For this review, take the finished solid that the model builds, in its own axes (mm). Face numbers are marked on the shaded views. A direction names the side the tool comes from. Coordinates: 2 decimals unless noted, no trailing zeros. Write each loop counter-clockwise with the first axis right and the second up, starting at its lowest first coordinate (ties: lowest second). Pieces come first, ordered by that corner, then holes. Notation, with made-up numbers: (-8.75, 66.5) - (38.25, 66.5) arc R15 cw to (38.25, 93.5) - close; hole circle Ø4 at (-37, 3.25). An arc over 180 degrees is marked (long way). Write each question's results on one line, items separated by ' | '.
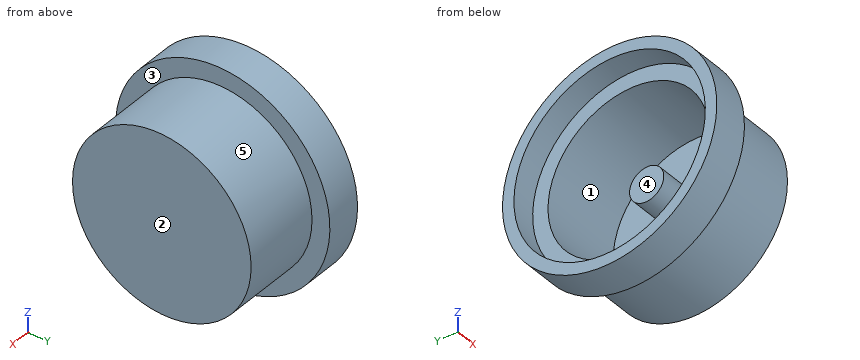
from build123d import *

# Parameters (mm, degrees)
SPUR_START             = 15.199213342
SPUR_GEAR_AM_OUTLINE_R = 1.5
SPUR_GEAR_AM_DEPTH     = 12
SKETCH9_R              = 1.5
BOSS_EXTRUDE1_DEPTH    = 12
SKETCH10_R             = 2.874
BOSS_EXTRUDE2_DEPTH    = 10
SKETCH11_R             = 15
BOSS_EXTRUDE3_DEPTH    = 1
SKETCH12_R             = 15
SKETCH12_R_2           = 13.5
BOSS_EXTRUDE4_DEPTH    = 13
SKETCH13_R             = 18
SKETCH13_R_2           = 13.5
BOSS_EXTRUDE5_DEPTH    = 1.9
SKETCH14_R             = 18
SKETCH14_R_2           = 16.075
BOSS_EXTRUDE6_DEPTH    = 4
SKETCH17_R             = 4
CUT_EXTRUDE2_DEPTH     = 41.416963439
SKETCH19_R             = 2.874
BOSS_EXTRUDE7_DEPTH    = 10


# Read off the part's stored shape, not the designer's step: spur gear_am
with BuildPart() as part:
    # spur gear_am outline → spur gear_am (new body)
    with BuildSketch(Plane.YZ.offset(SPUR_START)):
        with BuildLine():
            ThreePointArc((2.747947228, -4.643773619), (2.654088149, -4.687486435), (2.561391914, -4.733613923))
            ThreePointArc((2.561391914, -4.733613923), (2.561783739, -5.337982285), (2.816889806, -5.88587111))
            ThreePointArc((2.816889806, -5.88587111), (2.597713415, -6.044378226), (2.394409068, -6.222788256))
            ThreePointArc((2.394409068, -6.222788256), (1.9170234, -5.852161498), (1.327895004, -5.717294884))
            ThreePointArc((1.327895004, -5.717294884), (1.262297175, -5.797402699), (1.198794721, -5.879181519))
            ThreePointArc((1.198794721, -5.879181519), (1.461373347, -6.423528591), (1.928936024, -6.806472991))
            ThreePointArc((1.928936024, -6.806472991), (1.800238579, -7.04438004), (1.694476903, -7.293332374))
            ThreePointArc((1.694476903, -7.293332374), (1.103558354, -7.166539081), (0.514255579, -7.300641692))
            ThreePointArc((0.514255579, -7.300641692), (0.489911456, -7.401278171), (0.468180222, -7.502511024))
            ThreePointArc((0.468180222, -7.502511024), (0.940938733, -7.879022193), (1.528351497, -8.021175333))
            ThreePointArc((1.528351497, -8.021175333), (1.515623105, -8.291361907), (1.528351497, -8.56154848))
            ThreePointArc((1.528351497, -8.56154848), (0.940938733, -8.70370162), (0.468180222, -9.080212789))
            ThreePointArc((0.468180222, -9.080212789), (0.489911456, -9.181445642), (0.514255579, -9.28208212))
            ThreePointArc((0.514255579, -9.28208212), (1.103558354, -9.416184732), (1.694476903, -9.289391439))
            ThreePointArc((1.694476903, -9.289391439), (1.800238579, -9.538343772), (1.928936024, -9.776250821))
            ThreePointArc((1.928936024, -9.776250821), (1.461373347, -10.159195221), (1.198794721, -10.703542294))
            ThreePointArc((1.198794721, -10.703542294), (1.262297175, -10.785321114), (1.327895004, -10.865428928))
            ThreePointArc((1.327895004, -10.865428928), (1.9170234, -10.730562315), (2.394409068, -10.359935556))
            ThreePointArc((2.394409068, -10.359935556), (2.597713414, -10.538345587), (2.816889806, -10.696852703))
            ThreePointArc((2.816889806, -10.696852703), (2.561783739, -11.244741528), (2.561391914, -11.84910989))
            ThreePointArc((2.561391914, -11.84910989), (2.654088149, -11.895237378), (2.747947228, -11.938950194))
            ThreePointArc((2.747947228, -11.938950194), (3.220217142, -11.561826343), (3.489517843, -11.020773293))
            ThreePointArc((3.489517843, -11.020773293), (3.750097941, -11.093304726), (4.016342706, -11.14101763))
            ThreePointArc((4.016342706, -11.14101763), (4.024220134, -11.745334779), (4.286092716, -12.290021864))
            ThreePointArc((4.286092716, -12.290021864), (4.389623105, -12.291361906), (4.493153494, -12.290021864))
            ThreePointArc((4.493153494, -12.290021864), (4.755026076, -11.745334779), (4.762903504, -11.14101763))
            ThreePointArc((4.762903504, -11.14101763), (5.029148269, -11.093304726), (5.289728367, -11.020773293))
            ThreePointArc((5.289728367, -11.020773293), (5.559029068, -11.561826343), (6.031298982, -11.938950194))
            ThreePointArc((6.031298982, -11.938950194), (6.125158061, -11.895237378), (6.217854296, -11.84910989))
            ThreePointArc((6.217854296, -11.84910989), (6.217462471, -11.244741528), (5.962356404, -10.696852703))
            ThreePointArc((5.962356404, -10.696852703), (6.181532796, -10.538345587), (6.384837142, -10.359935556))
            ThreePointArc((6.384837142, -10.359935556), (6.86222281, -10.730562315), (7.451351206, -10.865428928))
            ThreePointArc((7.451351206, -10.865428928), (7.516949035, -10.785321114), (7.580451489, -10.703542294))
            ThreePointArc((7.580451489, -10.703542294), (7.317872863, -10.159195221), (6.850310186, -9.776250821))
            ThreePointArc((6.850310186, -9.776250821), (6.979007631, -9.538343772), (7.084769307, -9.289391439))
            ThreePointArc((7.084769307, -9.289391439), (7.675687856, -9.416184732), (8.26499063, -9.28208212))
            ThreePointArc((8.26499063, -9.28208212), (8.289334754, -9.181445642), (8.311065988, -9.080212789))
            ThreePointArc((8.311065988, -9.080212789), (7.838307477, -8.70370162), (7.250894713, -8.56154848))
            ThreePointArc((7.250894713, -8.56154848), (7.263623105, -8.291361907), (7.250894713, -8.021175333))
            ThreePointArc((7.250894713, -8.021175333), (7.838307477, -7.879022193), (8.311065988, -7.502511024))
            ThreePointArc((8.311065988, -7.502511024), (8.289334754, -7.40127817), (8.26499063, -7.300641692))
            ThreePointArc((8.26499063, -7.300641692), (7.675687856, -7.166539081), (7.084769307, -7.293332374))
            ThreePointArc((7.084769307, -7.293332374), (6.979007631, -7.04438004), (6.850310186, -6.806472991))
            ThreePointArc((6.850310186, -6.806472991), (7.317872863, -6.423528591), (7.580451489, -5.879181519))
            ThreePointArc((7.580451489, -5.879181519), (7.516949035, -5.797402699), (7.451351206, -5.717294884))
            ThreePointArc((7.451351206, -5.717294884), (6.86222281, -5.852161498), (6.384837142, -6.222788256))
            ThreePointArc((6.384837142, -6.222788256), (6.181532795, -6.044378226), (5.962356404, -5.88587111))
            ThreePointArc((5.962356404, -5.88587111), (6.217462471, -5.337982285), (6.217854296, -4.733613923))
            ThreePointArc((6.217854296, -4.733613923), (6.125158061, -4.687486435), (6.031298982, -4.643773619))
            ThreePointArc((6.031298982, -4.643773619), (5.559029068, -5.02089747), (5.289728367, -5.56195052))
            ThreePointArc((5.289728367, -5.56195052), (5.029148269, -5.489419087), (4.762903504, -5.441706183))
            ThreePointArc((4.762903504, -5.441706183), (4.755026076, -4.837389034), (4.493153494, -4.292701948))
            ThreePointArc((4.493153494, -4.292701948), (4.389623105, -4.291361906), (4.286092716, -4.292701948))
            ThreePointArc((4.286092716, -4.292701948), (4.024220134, -4.837389034), (4.016342706, -5.441706183))
            ThreePointArc((4.016342706, -5.441706183), (3.750097941, -5.489419087), (3.489517843, -5.56195052))
            ThreePointArc((3.489517843, -5.56195052), (3.220217142, -5.02089747), (2.747947228, -4.643773619))
        make_face()
        with Locations((4.389623105, -8.291361906)):
            Circle(SPUR_GEAR_AM_OUTLINE_R, mode=Mode.SUBTRACT)
    extrude(amount=SPUR_GEAR_AM_DEPTH)

    # Sketch9 → Boss-Extrude1 (add, through all)
    with BuildSketch(Plane(origin=(27.199213342, 0, 0), x_dir=(0, 0, -1), z_dir=(1, 0, 0))):
        with Locations((8.291361906, 4.389623105)):
            Circle(SKETCH9_R)
    extrude(amount=-BOSS_EXTRUDE1_DEPTH)

    # Sketch10 → Boss-Extrude2 (add)
    with BuildSketch(Plane(origin=(27.199213342, 0, 0), x_dir=(0, 0, -1), z_dir=(1, 0, 0))):
        with Locations(Location((8.291361906, 4.389623105, 0), (0, 0, 172.537235833))):
            Circle(SKETCH10_R)
    extrude(amount=BOSS_EXTRUDE2_DEPTH)

    # Sketch11 → Boss-Extrude3 (add)
    with BuildSketch(Plane(origin=(37.199213342, 0, 0), x_dir=(0, 0, -1), z_dir=(1, 0, 0))):
        with Locations((8.291361906, 4.389623105)):
            Circle(SKETCH11_R)
    extrude(amount=-BOSS_EXTRUDE3_DEPTH)

    # Sketch12 → Boss-Extrude4 (add)
    with BuildSketch(Plane.ZY.offset(-37.199213342)):
        with Locations(Location((-8.291361906, 4.389623105, 0), (0, 0, 180))):
            Circle(SKETCH12_R)
        with Locations(Location((-8.291361906, 4.389623105, 0), (0, 0, 180))):
            Circle(SKETCH12_R_2, mode=Mode.SUBTRACT)
    extrude(amount=BOSS_EXTRUDE4_DEPTH)

    # Sketch13 → Boss-Extrude5 (add)
    with BuildSketch(Plane.ZY.offset(-24.199213342)):
        with Locations(Location((-8.291361906, 4.389623105, 0), (0, 0, 180))):
            Circle(SKETCH13_R)
        with Locations(Location((-8.291361906, 4.389623105, 0), (0, 0, 180))):
            Circle(SKETCH13_R_2, mode=Mode.SUBTRACT)
    extrude(amount=BOSS_EXTRUDE5_DEPTH)

    # Sketch14 → Boss-Extrude6 (add)
    with BuildSketch(Plane.ZY.offset(-22.299213342)):
        with Locations(Location((-8.291361906, 4.389623105, 0), (0, 0, 180))):
            Circle(SKETCH14_R)
        with Locations((-8.291361906, 4.389623105)):
            Circle(SKETCH14_R_2, mode=Mode.SUBTRACT)
    extrude(amount=BOSS_EXTRUDE6_DEPTH)

    # Sketch17 → Cut-Extrude2 (cut, through all)
    with BuildSketch(Plane.ZY.offset(-36.199213342)):
        with Locations((-8.291361906, 4.389623105)):
            Circle(SKETCH17_R)
    extrude(amount=CUT_EXTRUDE2_DEPTH, mode=Mode.SUBTRACT)

    # Sketch19 → Boss-Extrude7 (add)
    with BuildSketch(Plane.ZY.offset(-36.199213342)):
        with Locations(Location((-8.291361906, 4.389623105, 0), (0, 0, 180))):
            Circle(SKETCH19_R)
    extrude(amount=BOSS_EXTRUDE7_DEPTH)


solid = part.part
Q1. Take a section at A-A on x = 32.75. State the section outline as (y, z) points.
Results found:
outline: circle Ø30 at (4.39, -8.29); circle Ø5.75 at (4.39, -8.29); hole circle Ø27 at (4.39, -8.29)
Q2. Mouldability with a two-part tool opening along Y and no side actions: class the marked faces 3, 4 and 5 as pulls with the +Y half, pulls with the -Y half, needs draft (parallel to the pull), parting line crosses it, or undercut.
Results found:
face 3: needs draft | face 4: undercut | face 5: parting line crosses it
Q3. Take a section at D-D on x = 23.5. State the section outline as (y, z) points, plus the area to 3 significant figures.
Results found:
outline: circle Ø36 at (4.39, -8.29); hole circle Ø27 at (4.39, -8.29) | area: 445 mm2
Q4. Wall thickness on line 1 along Z through (x, y) = (35, 4.5); line 2 along Z through (x, y) = (27.5, 6); line 3 along Y through (x, z) = (27, -7): over which ranges is each line inside the solid? List them lowest first. Write a range as from..to.
Results found:
line 1: -23.29..-21.79, -11.16..-5.42, 5.21..6.71 | line 2: -23.2..-21.69, -10.67..-5.91, 5.11..6.62 | line 3: -10.55..-9.05, 1.82..6.96, 17.83..19.33
Q5. For the marked faces 1 and 2, list the 3-axis set-ups (+Z, -Z, +X, -X, +Y, -Y) from which the entire face can be reached by the end or side of a thin tool; tool diameter is ignored.
Results found:
face 1: -X | face 2: +Z, -Z, +X, +Y, -Y
Q6. For pin 1 (2 mm diameter, centred on x = 27, y = 18.5, fed in from -Z); pin 2 (2 mm diameter, centred on x = 21.5, z = 5, fed in from +Y); pin 3 (6 mm diameter, centred on x = 21.5, z = -9, fed in from +Y), all flat-tipped, find the tip position at first contact; note any pin that passes through.
Results found:
pin 1: z = -15.58 | pin 2: y = 17.54 | pin 3: y = 22.39
Q7. Take a section at B-B on y = -1.5. State the section outline as (x, z) points, plus the area to 3 significant figures.
Results found:
outline: (18.3, -25.3) - (24.2, -25.3) - (24.2, -22.09) - (37.2, -22.09) - (37.2, 5.5) - (24.2, 5.5) - (24.2, 8.72) - (18.3, 8.72) - (18.3, 6.67) - (22.3, 6.67) - (22.3, 3.86) - (36.2, 3.86) - (36.2, -20.44) - (22.3, -20.44) - (22.3, -23.25) - (18.3, -23.25) - close | area: 102 mm2
Q8. Take a section at C-C on z = -14. State the section outline as (x, y) points, plus the area to 3 significant figures.
Results found:
outline: (18.3, -12.68) - (24.2, -12.68) - (24.2, -9.48) - (37.2, -9.48) - (37.2, 18.26) - (24.2, 18.26) - (24.2, 21.46) - (18.3, 21.46) - (18.3, 19.42) - (22.3, 19.42) - (22.3, 16.62) - (36.2, 16.62) - (36.2, -7.84) - (22.3, -7.84) - (22.3, -10.64) - (18.3, -10.64) - close | area: 102 mm2
